```python
from build123d import *

# Parameters (mm, degrees)
CROQUIS1_R              = 2
CROQUIS1_R_2            = 4
CROQUIS1_R_3            = 1.5
SALIENTE_EXTRUIR1_DEPTH = 4
REDONDEO1_R             = 10


with BuildPart() as part:
    # Croquis1 → Saliente-Extruir1 (new body)
    with BuildSketch(Plane(origin=(0, 0, 0), x_dir=(1, 0, 0), z_dir=(0, 1, 0))):
        with BuildLine():
            Line((-42.5, 24.539487758), (-134.423881554, 116.463369312))
            Line((-134.423881554, 116.463369312), (-144.318030777, 117.91451064))
            Line((-144.318030777, 117.91451064), (-152.860628735, 124.671679333))
            ThreePointArc((-152.860628735, 124.671679333), (-156.639963967, 131.934164505), (-153.727896681, 139.585761057))
            Line((-153.727896681, 139.585761057), (-139.585761057, 153.727896681))
            ThreePointArc((-139.585761057, 153.727896681), (-131.934164505, 156.639963967), (-124.671679333, 152.860628735))
            Line((-124.671679333, 152.860628735), (-117.91451064, 144.318030777))
            Line((-117.91451064, 144.318030777), (-116.463369312, 134.423881554))
            Line((-116.463369312, 134.423881554), (-42.943057454, 60.903569696))
            Line((-42.943057454, 60.903569696), (-20, 93.669651468))
            Line((-20, 93.669651468), (20, 93.669651468))
            Line((20, 93.669651468), (42.943057454, 60.903569696))
            Line((42.943057454, 60.903569696), (116.463369312, 134.423881554))
            Line((116.463369312, 134.423881554), (117.91451064, 144.318030777))
            Line((117.91451064, 144.318030777), (124.671679333, 152.860628735))
            ThreePointArc((124.671679333, 152.860628735), (131.934164505, 156.639963967), (139.585761057, 153.727896681))
            Line((139.585761057, 153.727896681), (153.727896681, 139.585761057))
            ThreePointArc((153.727896681, 139.585761057), (156.639963967, 131.934164505), (152.860628735, 124.671679333))
            Line((152.860628735, 124.671679333), (144.318030777, 117.91451064))
            Line((144.318030777, 117.91451064), (134.423881554, 116.463369312))
            Line((134.423881554, 116.463369312), (42.5, 24.539487758))
            Line((42.5, 24.539487758), (42.5, -24.539487758))
            Line((42.5, -24.539487758), (134.423881554, -116.463369312))
            Line((134.423881554, -116.463369312), (144.318030777, -117.91451064))
            Line((144.318030777, -117.91451064), (152.860628735, -124.671679333))
            ThreePointArc((152.860628735, -124.671679333), (156.639963967, -131.934164505), (153.727896681, -139.585761057))
            Line((153.727896681, -139.585761057), (139.585761057, -153.727896681))
            ThreePointArc((139.585761057, -153.727896681), (131.934164505, -156.639963967), (124.671679333, -152.860628735))
            Line((124.671679333, -152.860628735), (117.91451064, -144.318030777))
            Line((117.91451064, -144.318030777), (116.463369312, -134.423881554))
            Line((116.463369312, -134.423881554), (42.5, -60.460512242))
            Line((42.5, -60.460512242), (42.5, -75.460512242))
            Line((42.5, -75.460512242), (32.5, -102.935286437))
            Line((32.5, -102.935286437), (-32.5, -102.935286437))
            Line((-32.5, -102.935286437), (-42.5, -75.460512242))
            Line((-42.5, -75.460512242), (-42.5, -60.460512242))
            Line((-42.5, -60.460512242), (-116.463369312, -134.423881554))
            Line((-116.463369312, -134.423881554), (-117.91451064, -144.318030777))
            Line((-117.91451064, -144.318030777), (-124.671679333, -152.860628735))
            ThreePointArc((-124.671679333, -152.860628735), (-131.934164505, -156.639963967), (-139.585761057, -153.727896681))
            Line((-139.585761057, -153.727896681), (-153.727896681, -139.585761057))
            ThreePointArc((-153.727896681, -139.585761057), (-156.639963967, -131.934164505), (-152.860628735, -124.671679333))
            Line((-152.860628735, -124.671679333), (-144.318030777, -117.91451064))
            Line((-144.318030777, -117.91451064), (-134.423881554, -116.463369312))
            Line((-134.423881554, -116.463369312), (-42.5, -24.539487758))
            Line((-42.5, -24.539487758), (-42.5, 24.539487758))
        make_face()
        with Locations((-127.870144559, 127.870144559)):
            Circle(CROQUIS1_R, mode=Mode.SUBTRACT)
        with Locations((-126.809484388, 140.24451323)):
            Circle(CROQUIS1_R, mode=Mode.SUBTRACT)
        with Locations((-140.24451323, 126.809484388)):
            Circle(CROQUIS1_R, mode=Mode.SUBTRACT)
        with Locations((-139.183853058, 139.183853058)):
            Circle(CROQUIS1_R, mode=Mode.SUBTRACT)
        with Locations((140.24451323, 126.809484388)):
            Circle(CROQUIS1_R, mode=Mode.SUBTRACT)
        with Locations((127.870144559, 127.870144559)):
            Circle(CROQUIS1_R, mode=Mode.SUBTRACT)
        with Locations((126.809484388, 140.24451323)):
            Circle(CROQUIS1_R, mode=Mode.SUBTRACT)
        with Locations((139.183853058, 139.183853058)):
            Circle(CROQUIS1_R, mode=Mode.SUBTRACT)
        with Locations((126.809484388, -140.24451323)):
            Circle(CROQUIS1_R, mode=Mode.SUBTRACT)
        with Locations((127.870144559, -127.870144559)):
            Circle(CROQUIS1_R, mode=Mode.SUBTRACT)
        with Locations((140.24451323, -126.809484388)):
            Circle(CROQUIS1_R, mode=Mode.SUBTRACT)
        with Locations((139.183853058, -139.183853058)):
            Circle(CROQUIS1_R, mode=Mode.SUBTRACT)
        with Locations((-140.24451323, -126.809484388)):
            Circle(CROQUIS1_R, mode=Mode.SUBTRACT)
        with Locations((-127.870144559, -127.870144559)):
            Circle(CROQUIS1_R, mode=Mode.SUBTRACT)
        with Locations((-126.809484388, -140.24451323)):
            Circle(CROQUIS1_R, mode=Mode.SUBTRACT)
        with Locations((-139.183853058, -139.183853058)):
            Circle(CROQUIS1_R, mode=Mode.SUBTRACT)
        with Locations((32.5, -75.460512242)):
            Circle(CROQUIS1_R, mode=Mode.SUBTRACT)
        with Locations((-32.5, -75.460512242)):
            Circle(CROQUIS1_R, mode=Mode.SUBTRACT)
        with Locations((-32.5, 60.907651634)):
            Circle(CROQUIS1_R, mode=Mode.SUBTRACT)
        with Locations((32.5, 60.907651634)):
            Circle(CROQUIS1_R, mode=Mode.SUBTRACT)
        with Locations((-32.5, -7.276430304)):
            Circle(CROQUIS1_R, mode=Mode.SUBTRACT)
        with Locations((32.5, -7.276430304)):
            Circle(CROQUIS1_R, mode=Mode.SUBTRACT)
        with Locations((-133.526998809, 133.526998809)):
            Circle(CROQUIS1_R_2, mode=Mode.SUBTRACT)
        with Locations((133.526998809, 133.526998809)):
            Circle(CROQUIS1_R_2, mode=Mode.SUBTRACT)
        with Locations((133.526998809, -133.526998809)):
            Circle(CROQUIS1_R_2, mode=Mode.SUBTRACT)
        with Locations((-133.526998809, -133.526998809)):
            Circle(CROQUIS1_R_2, mode=Mode.SUBTRACT)
        with Locations((15.25, 15.25)):
            Circle(CROQUIS1_R_3, mode=Mode.SUBTRACT)
        with Locations((15.25, -15.25)):
            Circle(CROQUIS1_R_3, mode=Mode.SUBTRACT)
        with Locations((-15.25, -15.25)):
            Circle(CROQUIS1_R_3, mode=Mode.SUBTRACT)
        with Locations((-15.25, 15.25)):
            Circle(CROQUIS1_R_3, mode=Mode.SUBTRACT)
    extrude(amount=SALIENTE_EXTRUIR1_DEPTH)

    # Redondeo1
    redondeo1_edges = [part.edges().sort_by_distance(p)[0] for p in [
        (32.5, 2, 102.935286437),
        (-32.5, 2, 102.935286437),
    ]]
    fillet(redondeo1_edges, radius=REDONDEO1_R)


solid = part.part
```
Geometry check sheet. Reference: the model listing, model coordinates, mm. A direction names the side the tool comes from. Give positions to 0.01 mm unless a question says otherwise; leave off trailing zeros. Order: outer loops, then holes, each group sorted by start corner. A loop starts at its lowest first (then second) coordinate and runs counter-clockwise, first axis right, second up.
1. Release check for a two-part mould opening along Z. For faces 1 (the face through (1, 4, -12)), 2 (the face through (31.31, 1.97, -77.52)), 3 (the face through (148.6, 2, -121.3)) record: pulls with the +Z half, pulls with the -Z half, needs draft (parallel to the pull), parting line crosses it, or undercut.
2. Section check B-B, the plane x = 74. Enter the section's corners in (y, z), and give its area (3 significant figures).
3. Section check A-A, the plane z = 83.5. Enter the section's corners in (x, y).
4. Thickness scan on L1, parallel to Z at x = 15.25, y = 1.55; L2, parallel to X at y = 3.7, z = -125; L3, parallel to X at y = 2, z = 14.5. Record the ranges inside material, lowest first.
5. Gauge pin test, flat ends, axial feed: pin 1 Ø1 at (y, z) = (2, -90) entering from +X; pin 2 Ø2 at (x, y) = (62.5, 1.5) entering from +Z; pin 3 Ø2.5 at (x, z) = (-15.25, -15.25) entering from -Y; pin 4 Ø2 at (x, y) = (94, 0.5) entering from +Z. Record the tip position at first contact, or that the pin passes through.
6. Section check D-D, the plane y = 0.6. Give the number of separate pieces and of enclosed holes in the cut face, and give its area (3 significant figures).
7. Access from +Z, -Z, +X, -X, +Y, -Y to the whole of each face (thin tool, end or side, straight path). Record for faces 4 (the face through (121.3, 2, 148.6)), 5 (the face through (-89.105, 1.972, 71.145)), 6 (the face through (-137.523, 1.972, -133.703)), 7 (the face through (-31.6, 2, -77.1)).
8. Section check C-C, the plane z = -9. Enter the section's corners in (x, y).
Values follow:
1. face 1: needs draft
1. face 2: pulls with the -Z half
1. face 3: undercut
2. outline: (0, -91.96) - (4, -91.96) - (4, -56.04) - (0, -56.04) - close; (0, 56.04) - (4, 56.04) - (4, 91.96) - (0, 91.96) - close
2. area: 287 mm2
3. outline: (-101.46, 0) - (-65.54, 0) - (-65.54, 4) - (-101.46, 4) - close; (-39.57, 0) - (39.57, 0) - (39.57, 4) - (-39.57, 4) - close; (65.54, 0) - (101.46, 0) - (101.46, 4) - (65.54, 4) - close
4. L1: z = -93.67 to -16.75, -13.75 to 13.75, 16.75 to 102.94
4. L2: x = -153.25 to -141.1, -139.39 to -107.04, 107.04 to 139.39, 141.1 to 153.25
4. L3: x = -42.5 to -16.55, -13.95 to 13.95, 16.55 to 42.5
5. pin 1: stops at x = 108.46
5. pin 2: stops at z = 81.46
5. pin 3: passes through
5. pin 4: stops at z = 112.96
6. separate pieces: 1
6. enclosed holes: 30
6. area: 31,400 mm2
7. face 4: +Z, +Y, -Y
7. face 5: -X, +Y, -Y
7. face 6: +Y, -Y
7. face 7: -Z, +Y, -Y
8. outline: (-42.5, 0) - (42.5, 0) - (42.5, 4) - (-42.5, 4) - close
